```python
from build123d import *

# Parameters (mm, degrees)
SKETCH1_R           = 60
BOSS_EXTRUDE1_DEPTH = 100
SHELL1_T            = -5
SKETCH3_R           = 32.5
CUT_EXTRUDE1_DEPTH  = 132.148770486
SKETCH4_R           = 5
CUT_EXTRUDE2_DEPTH  = 132.148770486


with BuildPart() as part:
    # Sketch1 → Boss-Extrude1 (new body)
    with BuildSketch(Plane(origin=(0, 0, 0), x_dir=(1, 0, 0), z_dir=(0, 1, 0))):
        with Locations(Location((0, 0, 0), (0, 0, 270))):
            Circle(SKETCH1_R)
    extrude(amount=BOSS_EXTRUDE1_DEPTH)

    # Shell1
    shell1_openings = [part.faces().sort_by_distance(p)[0] for p in [
        (0, 0, 0),
    ]]
    offset(amount=SHELL1_T, openings=shell1_openings, kind=Kind.INTERSECTION)

    # Sketch3 → Cut-Extrude1 (cut, through all)
    with BuildSketch(Plane(origin=(0, 100, 0), x_dir=(1, 0, 0), z_dir=(0, 1, 0))):
        with Locations(Location((0, 0, 0), (0, 0, 270))):
            Circle(SKETCH3_R)
    extrude(amount=-CUT_EXTRUDE1_DEPTH, mode=Mode.SUBTRACT)

    # Sketch4 → Cut-Extrude2 (cut, through all)
    with BuildSketch(Plane(origin=(0, 100, 0), x_dir=(1, 0, 0), z_dir=(0, 1, 0))):
        with Locations(Location((45, 0, 0), (0, 0, 270))):
            Circle(SKETCH4_R)
        with Locations(Location((-45, 0, 0), (0, 0, 270))):
            Circle(SKETCH4_R)
    extrude(amount=-CUT_EXTRUDE2_DEPTH, mode=Mode.SUBTRACT)


solid = part.part
```
Read the model definition and answer for the solid it produces. Units are mm, in the model's axes. A direction names the side the tool comes from. Coordinates: 2 decimals unless noted, no trailing zeros. Write each loop counter-clockwise with the first axis right and the second up, starting at its lowest first coordinate (ties: lowest second). Pieces come first, ordered by that corner, then holes. Notation, with made-up numbers: (25, 38.5) - (30, 38.5) arc R15 ccw to (30, 61.5) - close; hole circle Ø2 at (70.5, 73). An arc over 180 degrees is marked (long way). Answer as a JSON object with one key per item and string values. Group by question number.
1. A cutting plane is placed at D-D (z = -19.5). Determine the outline of the cut face in (x, y), plus the area to 3 significant figures.
2. A cutting plane is placed at C-C (y = 92). Determine the outline of the cut face in (x, z), plus the area to 3 significant figures.
3. The mould has two halves that part along Z. Classify faces 1 (the cylindrical face through (49.957, 97.535, -0.651)), 2 (the flat face through (-26, 100, 26)), 3 (the cylindrical face through (2.64, 49.3, -59.94)): +Z half, -Z half, draft (parallel to the pull), parting line (faces both ways), or undercut.
4. Consider L1, parallel to X at y = 97, z = 0; L2, parallel to X at y = 43, z = 1; L3, parallel to Y at x = 2.5, z = 34.5. Determine where each line is inside the solid, lowest interval first. Write a range as [from, to].
5. A cutting plane is placed at A-A (x = 0). Determine the outline of the cut face in (y, z), plus the area to 4 significant figures.
6. A cutting plane is placed at B-B (z = 0). Determine the outline of the cut face in (x, y).
7. Each of these flat-tipped pins is pushed along its axis until it touches: P1, Ø10, axis at y = 43.5, z = 39.5, coming from the -X side; P2, Ø8, axis at x = 41.5, z = -23.5, coming from the -Y side; P3, Ø3, axis at x = -7, y = 38.5, coming from the -Z side. Where does it stop, or does it pass through?
8. Which of the six approach directions +Z, -Z, +X, -X, +Y, -Y give full straight-line access (tool end or side, diameter ignored) to faces 4 (the flat face through (-24, 95, 24)), 5 (the cylindrical face through (-40.043, 97.535, -0.651))?
Worked out:
{
 "1": {"outline": "(-56.74, 0) - (-51.43, 0) - (-51.43, 95) - (-26, 95) - (-26, 100) - (-56.74, 100) - close; (26, 95) - (51.43, 95) - (51.43, 0) - (56.74, 0) - (56.74, 100) - (26, 100) - close", "area": "1,320 mm²"},
 "2": {"outline": "circle Ø120 at (0, 0); hole circle Ø110 at (0, 0)", "area": "1,810 mm²"},
 "3": {"face 1": "undercut", "face 2": "draft", "face 3": "parting line"},
 "4": {"L1": "x = [-60, -50], [-40, -32.5], [32.5, 40], [50, 60]", "L2": "x = [-59.99, -54.99], [54.99, 59.99]", "L3": "y = [95, 100]"},
 "5": {"outline": "(0, -60) - (100, -60) - (100, -32.5) - (95, -32.5) - (95, -55) - (0, -55) - close; (0, 55) - (95, 55) - (95, 32.5) - (100, 32.5) - (100, 60) - (0, 60) - close", "area": "1,225 mm²"},
 "6": {"outline": "(-60, 0) - (-55, 0) - (-55, 95) - (-50, 95) - (-50, 100) - (-60, 100) - close; (-40, 95) - (-32.5, 95) - (-32.5, 100) - (-40, 100) - close; (32.5, 95) - (40, 95) - (40, 100) - (32.5, 100) - close; (50, 95) - (55, 95) - (55, 0) - (60, 0) - (60, 100) - (50, 100) - close"},
 "7": {"P1": "stops at x = -49.09", "P2": "stops at y = 95", "P3": "stops at z = -59.75"},
 "8": {"face 4": "-Y", "face 5": "+Y, -Y"}
}
